Build history of the part. All positions in model axes, mm. A direction names the side the tool comes from. Round coordinates to 2 decimals unless told otherwise and drop trailing zeros. Order: outer loops, then holes, each group sorted by start corner. A loop starts at its lowest first (then second) coordinate and runs counter-clockwise, first axis right, second up. Notation, with made-up numbers: (28, 3.5) - (63, 3.5) arc R34 cw to (63, 33.5) - close; hole circle Ø10 at (37.25, 16). An arc over 180 degrees is marked (long way). Write each question's results on one line, items separated by ' | '. Start each with the question number.
```python
from build123d import *

# Parameters (mm, degrees)
EXTRUDE_1_DEPTH     = 8
SKETCH_2_R          = 2
CUT_EXTRUDE_1_DEPTH = 15
SKETCH_3_R          = 2
CUT_EXTRUDE_2_DEPTH = 15
FILLET_1_R          = 2


with BuildPart() as part:
    # 草图1 → 凸台-拉伸1 (new body)
    with BuildSketch(Plane.XY):
        with BuildLine():
            Line((-15, 0), (-15, -25))
            Line((-15, -25), (-15, -40))
            Line((-15, -40), (15, -40))
            Line((15, -40), (15, 0))
            ThreePointArc((15, 0), (14.624937393, 3.333347603), (13.518505835, 6.5))
            Line((13.518505835, 6.5), (7, 6.5))
            Line((7, 6.5), (7, 13.266499161))
            ThreePointArc((7, 13.266499161), (4.089328898, 14.431818637), (1, 14.966629547))
            Line((1, 14.966629547), (1, 4.898979486))
            ThreePointArc((1, 4.898979486), (4.878315178, 1.096376317), (3, -4))
            Line((3, -4), (-3, -4))
            ThreePointArc((-3, -4), (-4.878315178, 1.096376317), (-1, 4.898979486))
            Line((-1, 4.898979486), (-1, 14.966629547))
            ThreePointArc((-1, 14.966629547), (-4.089328898, 14.431818637), (-7, 13.266499161))
            Line((-7, 13.266499161), (-7, 6.5))
            Line((-7, 6.5), (-13.518505835, 6.5))
            ThreePointArc((-13.518505835, 6.5), (-14.624937393, 3.333347603), (-15, 0))
        make_face()
    extrude(amount=EXTRUDE_1_DEPTH)

    # 草图2 → 切除-拉伸1 (cut)
    with BuildSketch(Plane(origin=(7, 0, 0), x_dir=(0, 0, -1), z_dir=(1, 0, 0))):
        with Locations((-4, 9.883249581)):
            Circle(SKETCH_2_R)
    extrude(amount=-CUT_EXTRUDE_1_DEPTH, mode=Mode.SUBTRACT)

    # 草图3 → 切除-拉伸2 (cut)
    with BuildSketch(Plane.XY.offset(8)):
        with Locations((7.5, -19)):
            Circle(SKETCH_3_R)
        with Locations((7.5, -33)):
            Circle(SKETCH_3_R)
        with Locations((-7.5, -33)):
            Circle(SKETCH_3_R)
        with Locations((-7.5, -19)):
            Circle(SKETCH_3_R)
    extrude(amount=-CUT_EXTRUDE_2_DEPTH, mode=Mode.SUBTRACT)

    # 圆角1
    fillet_1_edges = [part.edges().sort_by_distance(p)[0] for p in [
        (-13.518505835, 6.5, 4),
        (13.518505835, 6.5, 4),
        (15, -40, 4),
        (-15, -40, 4),
    ]]
    fillet(fillet_1_edges, radius=FILLET_1_R)


solid = part.part
```
1. Mould opens along Y. For faces 1 (the face through (4.86, 1.17, 3.94)), 2 (the face through (-14.76, 2.67, 3.94)), 3 (the face through (0, -12, 8)) say: pulls with the +Y half, pulls with the -Y half, needs draft (parallel to the pull), parting line crosses it, or undercut.
2. 3-axis set-ups, long thin cutter, end or side, ignore diameter. For faces 4 (the face through (-1, 9, 6)), 5 (the face through (10, 6.5, 4)), 6 (the face through (-10, 6.5, 4)), 7 (the face through (-4.9, 1, 3.9)): which of +Z, -Z, +X, -X, +Y, -Y reach the whole face in a straight line?
3. Cut at D-D (x = 6.25). List the corners of the cut face in (y, z).
4. Flat gauge pins, fed straight in: pin 1 Ø2.5 at (y, z) = (10, 3.5) entering from +X; pin 2 Ø1.5 at (x, z) = (-3, 3) entering from +Y; pin 3 Ø2.5 at (x, z) = (9.5, 5) entering from +Y; pin 4 Ø1.5 at (y, z) = (8, 3) entering from +X. Where does each tip first touch, or does it go through?
5. Wall check: line 1 (Y direction, x = 7.5, z = 2); line 2 (Y direction, x = 6.5, z = 4.25); line 3 (Y direction, x = -3.7, z = 4). Give the ranges that are in metal, low to high. Write a range as from..to.
6. Cut at B-B (x = 2). List the corners of the cut face in (y, z), plus the area to 3 significant figures.
7. Cut at C-C (y = -19). List the corners of the cut face in (x, z).
8. Cut at A-A (z = 4). Give the number of separate pieces and of enclosed holes in the cut face, plus the area to 3 significant figures.
A:
1) face 1: undercut | face 2: pulls with the +Y half | face 3: needs draft
2) face 4: +Z, -Z, +Y | face 5: +Z, -Z, +X, +Y | face 6: +Z, -Z, -X, +Y | face 7: +Z, -Z
3) outline: (-40, 0) - (-34.56, 0) - (-34.56, 8) - (-40, 8) - close; (-31.44, 0) - (-20.56, 0) - (-20.56, 8) - (-31.44, 8) - close; (-17.44, 0) - (13.64, 0) - (13.64, 8) - (-17.44, 8) - close; hole circle Ø4 at (9.88, 4)
4) pin 1: passes through | pin 2: stops at y = 14.83 | pin 3: stops at y = 6.5 | pin 4: stops at x = 7
5) line 1: y = -40..-35, -31..-21, -17..6.5 | line 2: y = -40..-34.73, -31.27..-20.73, -17.27..7.9, 11.87..13.52 | line 3: y = -40..-3.36, 3.36..7.88, 11.88..14.54
6) outline: (-40, 0) - (-4, 0) - (-4, 8) - (-40, 8) - close; (4.58, 0) - (14.87, 0) - (14.87, 8) - (4.58, 8) - close; hole circle Ø4 at (9.88, 4) | area: 358 mm^2
7) outline: (-15, 0) - (-9.5, 0) - (-9.5, 8) - (-15, 8) - close; (-5.5, 0) - (5.5, 0) - (5.5, 8) - (-5.5, 8) - close; (9.5, 0) - (15, 0) - (15, 8) - (9.5, 8) - close
8) separate pieces: 3 | enclosed holes: 4 | area: 1,300 mm^2
